Geometry check sheet. Reference: the model listing, model coordinates, mm. A direction names the side the tool comes from. Coordinates: 2 decimals unless noted, no trailing zeros. Order: outer loops, then holes, each group sorted by start corner. A loop starts at its lowest first (then second) coordinate and runs counter-clockwise, first axis right, second up. Notation, with made-up numbers: M 32,10 L 52,10 A23 cw 52,40 Z; hole C 82,66.25 d1. An arc over 180 degrees is marked long. One line per item, written item: value. Start each with the question number.
1) Sectioned sample at C-C, the plane z = -4.5. Enter the section's corners in (x, y), then the cut area to 3 significant figures.
2) Sectioned sample at A-A, the plane y = 0. Enter the section's corners in (x, z), then the cut area to 3 significant figures.
3) Sectioned sample at B-B, the plane z = 1.25. Enter the section's corners in (x, y).
4) Access from +Z, -Z, +X, -X, +Y, -Y to the whole of each face (thin tool, end or side, straight path). Record for faces 4 (the flat face through (-0.55, 4.36, 1.75)), 5 (the flat face through (-3.1, 0, -2)), 6 (the flat face through (4, 0, -5.5)).
5) Thickness scan on L1, parallel to Z at x = -6, y = -4; L2, parallel to X at y = 1.5, z = -1.25; L3, parallel to Y at x = 2.5, z = -4. Record the ranges inside material, lowest first. Write a range as from..to.
6) Go/stop test with flat-tipped pins: P1, Ø1.5, axis at x = 4, z = 0, coming from the +Y side; P2, Ø1.5, axis at x = 4.5, y = -6, coming from the -Z side; P3, Ø0.6, axis at x = 0.5, z = 2, coming from the -Y side; P4, Ø7.5, axis at x = -2, y = -3, coming from the -Z side. Record where each tip stops, or that it passes through.
7) Draft check along Y on faces 1 (the flat face through (3.1, 0, -2)), 2 (the flat face through (2, 6, 0)), 3 (the cylindrical face through (-6, 0, -2)). Enter one of: pulls with the +Y half, pulls with the -Y half, needs draft (parallel to the pull), parting line crosses it, or undercut.
```python
from build123d import *

# Parameters (mm, degrees)
SKETCH1_R           = 6
SKETCH1_W           = 6.2
SKETCH1_H           = 6.2
BOSS_EXTRUDE1_DEPTH = 5.5
BOSS_EXTRUDE2_START = 2
SKETCH1_3_R         = 8
SKETCH1_3_R_2       = 6
SKETCH1_3_W         = 6.2
SKETCH1_3_H         = 6.2
BOSS_EXTRUDE2_DEPTH = 2
FILLET1_R           = 0.5
CUT_EXTRUDE1_DEPTH  = 0.5


with BuildPart() as part:
    # Sketch1 → Boss-Extrude1 (new body)
    with BuildSketch(Plane.XY):
        Circle(SKETCH1_R)
        Rectangle(SKETCH1_W, SKETCH1_H, mode=Mode.SUBTRACT)
    extrude(amount=-BOSS_EXTRUDE1_DEPTH)

    # Sketch1_3 → Boss-Extrude2 (add)
    # profile 1 of 2: a face of its own
    with BuildSketch(Plane.XY.offset(BOSS_EXTRUDE2_START)):
        Circle(SKETCH1_3_R)
        Circle(SKETCH1_3_R_2, mode=Mode.SUBTRACT)
    # profile 2 of 2: a face of its own
    with BuildSketch(Plane.XY.offset(BOSS_EXTRUDE2_START)):
        Circle(SKETCH1_3_R_2)
        Rectangle(SKETCH1_3_W, SKETCH1_3_H, mode=Mode.SUBTRACT)
    extrude(amount=-BOSS_EXTRUDE2_DEPTH)

    # Fillet1
    fillet1_edges = [part.edges().sort_by_distance(p)[0] for p in [
        (-8, 0, 0),
        (-6, 0, -5.5),
    ]]
    fillet(fillet1_edges, radius=FILLET1_R)

    # Sketch2 → Cut-Extrude1 (cut)
    with BuildSketch(Plane.XY.offset(2)):
        with BuildLine():
            Line((-0.770976701, 6.067937408), (-1.085079266, 6.067937408))
            add(Edge.make_bspline(
                [(-1.085079266, 6.067937408), (-1.083032113, 6.109608296), (-1.079011558, 6.19144881), (-1.060183269, 6.310772717), (-1.033242392, 6.424827515), (-0.995150938, 6.532697429), (-0.94784466, 6.635336237), (-0.891114633, 6.732336252), (-0.823920782, 6.823327441), (-0.747714048, 6.907466284), (-0.664945409, 6.984653855), (-0.57563947, 7.051309098), (-0.481794442, 7.107626769), (-0.383695044, 7.154708011), (-0.28023448, 7.190047857), (-0.172351622, 7.216269497), (-0.059572486, 7.232045842), (0.017267536, 7.233741628), (0.056347017, 7.234604075)],
                knots=[0, 0, 0, 0, 1.10065271, 2.161652631, 3.183658789, 4.190468796, 5.17591951, 6.163126047, 7.15150782, 8.156236427, 9.156009102, 10.134482811, 11.092018607, 12.041330605, 13.001268258, 13.972401359, 14.968799086, 16, 16, 16, 16], degree=3))
            add(Edge.make_bspline(
                [(0.056347017, 7.234604075), (0.094725091, 7.233705618), (0.170136635, 7.231940183), (0.28019865, 7.216779154), (0.384975944, 7.193033562), (0.484263711, 7.159718146), (0.577269775, 7.114933719), (0.66469282, 7.06113618), (0.747573631, 6.998916349), (0.822180414, 6.925662535), (0.890688493, 6.847460151), (0.949790749, 6.763972247), (1.000403912, 6.677742961), (1.042591592, 6.58811476), (1.073647731, 6.494243731), (1.097225939, 6.397496529), (1.110553353, 6.296871718), (1.112598776, 6.228765162), (1.113638683, 6.194139331)],
                knots=[0, 0, 0, 0, 1.111607364, 2.184268762, 3.212621178, 4.221274766, 5.211760367, 6.196651075, 7.1921475, 8.207485113, 9.220403448, 10.201281604, 11.166441695, 12.114753415, 13.065576456, 14.026450734, 14.996634279, 16, 16, 16, 16], degree=3))
            add(Edge.make_bspline(
                [(1.113638683, 6.194139331), (1.11194542, 6.145391496), (1.108588609, 6.048751283), (1.079874232, 5.90673642), (1.035027721, 5.769143001), (0.981030364, 5.658405699), (0.92655792, 5.569172205), (0.877470413, 5.4957035), (0.820005602, 5.416598032), (0.753327104, 5.332120694), (0.678814232, 5.241609789), (0.595792068, 5.145119994), (0.503668586, 5.043648224), (0.439010086, 4.974342623), (0.40550567, 4.938430196)],
                knots=[0, 0, 0, 0, 1.184426356, 2.348067706, 3.509069118, 4.696110526, 5.333549288, 6.050745305, 6.844228056, 7.710549037, 8.667450064, 9.695053472, 10.805634456, 12, 12, 12, 12], degree=3))
            Line((0.40550567, 4.938430196), (-0.470195451, 4.003834844))
            Line((-0.470195451, 4.003834844), (1.158510478, 4.003834844))
            Line((1.158510478, 4.003834844), (1.158510478, 3.644860485))
            Line((1.158510478, 3.644860485), (-1.21969465, 3.644860485))
            Line((-1.21969465, 3.644860485), (0.137677145, 5.093378113))
            add(Edge.make_bspline(
                [(0.137677145, 5.093378113), (0.170725032, 5.12787642), (0.234203259, 5.194140606), (0.323985835, 5.290883566), (0.404624824, 5.380633107), (0.476642217, 5.463219656), (0.538475722, 5.539851223), (0.593347954, 5.608045927), (0.637313545, 5.670800377), (0.685028941, 5.743540991), (0.731242922, 5.832353308), (0.770955278, 5.940886998), (0.795170126, 6.05261425), (0.798074962, 6.128116287), (0.799536119, 6.166094459)],
                knots=[0, 0, 0, 0, 1.329631726, 2.553950428, 3.673215718, 4.687767853, 5.603093632, 6.413772471, 7.123043292, 7.734684054, 8.834405432, 9.900288307, 10.943827018, 12, 12, 12, 12], degree=3))
            add(Edge.make_bspline(
                [(0.799536119, 6.166094459), (0.798900377, 6.189975858), (0.797647451, 6.237041508), (0.786589753, 6.306047267), (0.769879247, 6.372612081), (0.745933989, 6.4369407), (0.714327249, 6.498386352), (0.675853869, 6.557023832), (0.631463806, 6.613712797), (0.580112536, 6.666866095), (0.523701017, 6.715547301), (0.464106767, 6.758671386), (0.401056663, 6.794710497), (0.334816541, 6.824253994), (0.265571071, 6.847429376), (0.193186326, 6.863487955), (0.11786231, 6.873570439), (0.066428814, 6.874934611), (0.040221215, 6.875629716)],
                knots=[0, 0, 0, 0, 0.991446411, 1.95395049, 2.89581595, 3.838931463, 4.798493298, 5.75982156, 6.748411868, 7.785213223, 8.824556874, 9.840280684, 10.836137867, 11.835679398, 12.848801643, 13.863922112, 14.911575587, 16, 16, 16, 16], degree=3))
            add(Edge.make_bspline(
                [(0.040221215, 6.875629716), (0.012850382, 6.874914683), (-0.040901414, 6.873510478), (-0.119820447, 6.863687814), (-0.195106224, 6.846741974), (-0.266948127, 6.823565299), (-0.335467713, 6.79410675), (-0.400331757, 6.757415006), (-0.461394646, 6.713631513), (-0.51877117, 6.663990956), (-0.571635149, 6.608723355), (-0.618082025, 6.547113392), (-0.658666039, 6.480285977), (-0.694075272, 6.408421426), (-0.722830962, 6.330867646), (-0.744804113, 6.247899941), (-0.762190959, 6.15987856), (-0.76799948, 6.099093475), (-0.770976701, 6.067937408)],
                knots=[0, 0, 0, 0, 1.031018746, 2.02475058, 2.990194455, 3.934040569, 4.864654155, 5.795059489, 6.735614925, 7.690564532, 8.649604399, 9.611025574, 10.590972636, 11.591080095, 12.624614302, 13.701020113, 14.821632451, 16, 16, 16, 16], degree=3))
        make_face()
    extrude(amount=-CUT_EXTRUDE1_DEPTH, mode=Mode.SUBTRACT)


solid = part.part
```
Final values:
1. outline: C 0,0 d12; hole M -3.1,-3.1 L 3.1,-3.1 L 3.1,3.1 L -3.1,3.1 Z
1. area: 74.7 mm^2
2. outline: M -8,0.5 A0.5 ccw -7.5,0 L -6,0 L -6,-5 A0.5 ccw -5.5,-5.5 L -3.1,-5.5 L -3.1,2 L -8,2 Z; M 3.1,-5.5 L 5.5,-5.5 A0.5 ccw 6,-5 L 6,0 L 7.5,0 A0.5 ccw 8,0.5 L 8,2 L 3.1,2 Z
2. area: 51.3 mm^2
3. outline: C 0,0 d16; hole M -3.1,-3.1 L 3.1,-3.1 L 3.1,3.1 L -3.1,3.1 Z
4. face 4: +Z
4. face 5: +Z, -Z
4. face 6: -Z, +X, -X, +Y, -Y
5. L1: z = 0..2
5. L2: x = -5.81..-3.1, 3.1..5.81
5. L3: y = -5.45..-3.1, 3.1..5.45
6. P1: stops at y = 7.25
6. P2: stops at z = 0
6. P3: stops at y = -8
6. P4: stops at z = -5.5
7. face 1: undercut
7. face 2: needs draft
7. face 3: parting line crosses it
